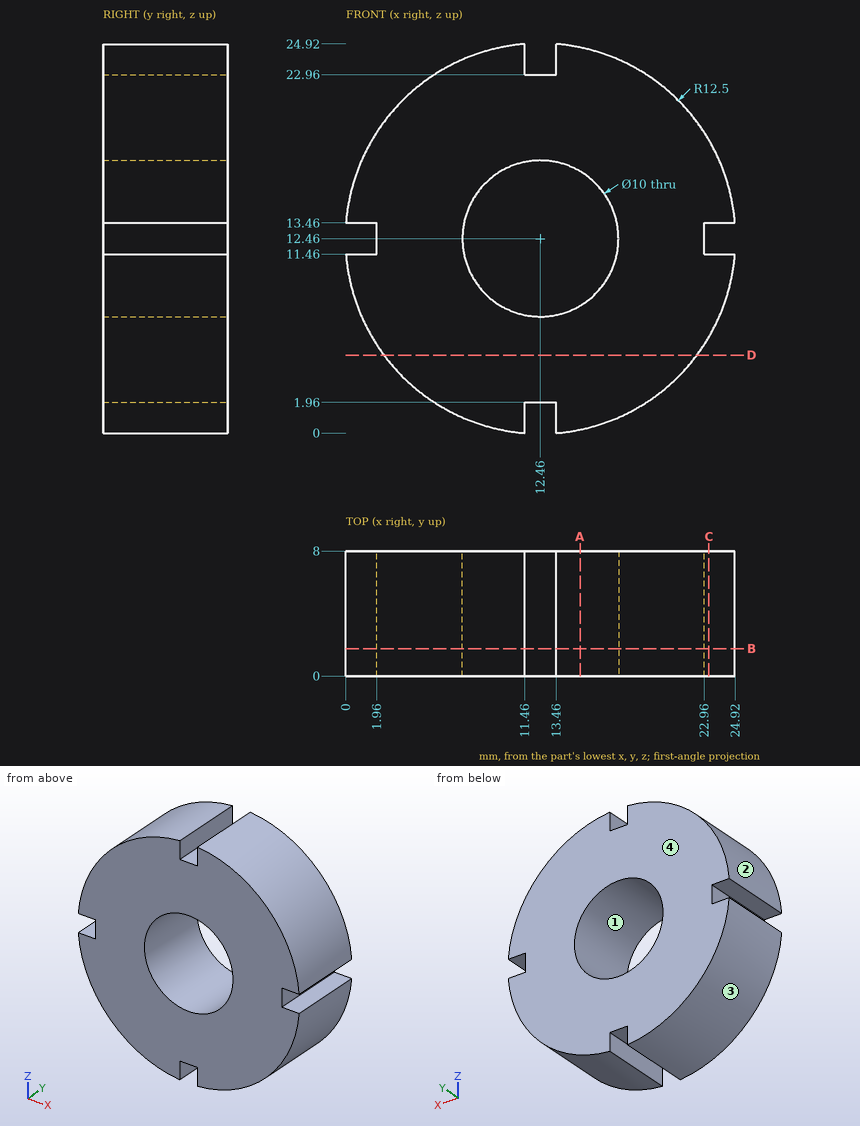
Part print with two shaded views. Sizes in mm from the minimum x, y, z corner. Coordinates: 2 decimals unless noted, no trailing zeros. Loops run counter-clockwise (first coordinate to the right, second up) from the corner with the lowest first, then second, coordinate; pieces in that order, holes last. Notation, with made-up numbers: (46, 41) - (64, 41) arc R9 ccw to (64, 53) - close; hole circle Ø7 at (8, 8.25). An arc over 180 degrees is marked (long way). Write each question's results on one line, items separated by ' | '. Start each with the question number.
Q1. Slice it at D-D on z = 5. Give the cut face in (x, y), and give its area (3 significant figures).
Q2. Slice it at C-C on x = 23.25. Give the cut face in (y, z), and give its area (3 significant figures).
Q3. Drop flat-ended pins along their axis: pin 1 Ø2 at (x, y) = (0.5, 4.5) entering from +Z; pin 2 Ø0.6 at (y, z) = (5.5, 1) entering from -X; pin 3 Ø2 at (y, z) = (3, 12.5) entering from -X; pin 4 Ø2 at (x, y) = (24, 2) entering from -Z. Give the stop position or say it passes through.
Q4. Two-plate mould, pull along Z, no slides. Class the marked faces 1, 2, 3 and 4: +Z half, -Z half, draft (parallel to the pull), parting line (faces both ways), or undercut.
Q5. Slice it at B-B on y = 1.75. Give the cut face in (x, z).
Q6. Slice it at A-A on x = 15. Give the cut face in (y, z).
Q7. Probe line 1 along X through (y, z) = (2.5, 23.75) (1 decimal); line 2 along X through (y, z) = (2, 23); line 3 along Z through (x, y) = (8.5, 1). List the from-to ranges inside material, lowest first.
Answer:
1) outline: (2.43, 0) - (22.49, 0) - (22.49, 8) - (2.43, 8) - close | area: 160 mm2
2) outline: (0, 6.15) - (8, 6.15) - (8, 11.46) - (0, 11.46) - close; (0, 13.46) - (8, 13.46) - (8, 18.77) - (0, 18.77) - close | area: 85.0 mm2
3) pin 1: stops at z = 18.47 | pin 2: stops at x = 6.83 | pin 3: stops at x = 0 | pin 4: stops at z = 5.74
4) face 1: undercut | face 2: +Z half | face 3: -Z half | face 4: draft
5) outline: (0, 11.46) arc R12.5 ccw to (11.46, 0) - (11.46, 1.96) - (13.46, 1.96) - (13.46, 0) arc R12.5 ccw to (24.92, 11.46) - (22.96, 11.46) - (22.96, 13.46) - (24.92, 13.46) arc R12.5 ccw to (13.46, 24.92) - (13.46, 22.96) - (11.46, 22.96) - (11.46, 24.92) arc R12.5 ccw to (0, 13.46) - (1.96, 13.46) - (1.96, 11.46) - close; hole circle Ø10 at (12.46, 12.46)
6) outline: (0, 0.22) - (8, 0.22) - (8, 8.15) - (0, 8.15) - close; (0, 16.77) - (8, 16.77) - (8, 24.7) - (0, 24.7) - close
7) line 1: x = 7.1 to 11.5, 13.5 to 17.8 | line 2: x = 5.74 to 11.46, 13.46 to 19.18 | line 3: z = 0.6 to 9.41, 15.51 to 24.32
